Could you check a few things on this model? Use its own coordinates, in mm. Face numbers are marked on the shaded views. A direction names the side the tool comes from. Coordinates: 2 decimals unless noted, no trailing zeros. Loops run counter-clockwise (first coordinate to the right, second up) from the corner with the lowest first, then second, coordinate; pieces in that order, holes last. Notation, with made-up numbers: (9.25, 84) -> (33.25, 84) arc R11 ccw to (33.25, 98) -> close; hole circle Ø8 at (31.5, -23.5). An arc over 180 degrees is marked (long way). One line per question, with ' | ' between items.
from build123d import *

# Parameters (mm, degrees)
SKETCH1_W                       = 9.5
SKETCH1_H                       = 3.26
BOSS_EXTRUDE1_DEPTH             = 11.42
BOSS_EXTRUDE3_REACH             = 14.475
BOSS_EXTRUDE3_DIRECTION_2_REACH = 14.475
FILLET1_R                       = 0.3
SKETCH4_R                       = 1.5
CUT_EXTRUDE1_DEPTH              = 16.081341077
FILLET2_R                       = 10


with BuildPart() as part:
    # Sketch1 → Boss-Extrude1 (new body)
    with BuildSketch(Plane.XY):
        Rectangle(SKETCH1_W, SKETCH1_H)
    extrude(amount=BOSS_EXTRUDE1_DEPTH)

    # Boss-Extrude3: up to this face of the body (flat: up to its plane)
    boss_extrude3_end = Plane(part.part.faces().sort_by_distance((-4.75, 0, 5.71))[0])
    # Sketch3 → Boss-Extrude3 (add, up to the picked face)
    with BuildSketch(Plane(origin=(0, 0, 0), x_dir=(0, 0, -1), z_dir=(1, 0, 0)), mode=Mode.PRIVATE) as boss_extrude3_sk1:
        with BuildLine():
            Line((0, -1.63), (5.2, -2.629157971))
            add(Edge.make_bspline(
                [(5.2, -2.629157971), (5.283052086, -2.547091023), (5.363844635, -2.459497383), (5.60978901, -2.164369944), (5.763042084, -1.936211317), (6.019426683, -1.436050674), (6.122353138, -1.164082205), (6.261824898, -0.594664263), (6.298216306, -0.297392436), (6.298215992, 0.297396341), (6.26182427, 0.594668129), (6.122351908, 1.164085924), (6.019425166, 1.436054284), (5.763040038, 1.936214656), (5.609786724, 2.164373121), (5.363842902, 2.459499262), (5.283051196, 2.547091902), (5.2, 2.629157971)],
                knots=[0.163498388, 0.163498388, 0.163498388, 0.163498388, 0.204239042, 0.204239042, 0.29258857, 0.29258857, 0.380938098, 0.380938098, 0.469287626, 0.469287626, 0.557637154, 0.557637154, 0.645986682, 0.645986682, 0.73433621, 0.73433621, 0.77507641, 0.77507641, 0.77507641, 0.77507641], degree=3))
            Line((5.2, 2.629157971), (0, 1.63))
            Line((0, 1.63), (0, -1.63))
        make_face()
    boss_extrude3_tool1 = split(extrude(boss_extrude3_sk1.sketch, amount=-BOSS_EXTRUDE3_REACH, mode=Mode.PRIVATE), bisect_by=boss_extrude3_end, keep=Keep.BOTH, mode=Mode.PRIVATE)
    add(boss_extrude3_tool1.solids().sort_by(Axis((0, 0, -3.236322), (-1, 0, 0)))[0])

    # Boss-Extrude3 direction 2: up to this face of the body (flat: up to its plane)
    boss_extrude3_direction_2_end = Plane(part.part.faces().sort_by_distance((4.75, 0, 5.71))[0])
    # Sketch3 → Boss-Extrude3 direction 2 (add, up to the picked face)
    with BuildSketch(Plane(origin=(0, 0, 0), x_dir=(0, 0, -1), z_dir=(1, 0, 0)), mode=Mode.PRIVATE) as boss_extrude3_direction_2_sk1:
        with BuildLine():
            Line((0, -1.63), (5.2, -2.629157971))
            add(Edge.make_bspline(
                [(5.2, -2.629157971), (5.283052086, -2.547091023), (5.363844635, -2.459497383), (5.60978901, -2.164369944), (5.763042084, -1.936211317), (6.019426683, -1.436050674), (6.122353138, -1.164082205), (6.261824898, -0.594664263), (6.298216306, -0.297392436), (6.298215992, 0.297396341), (6.26182427, 0.594668129), (6.122351908, 1.164085924), (6.019425166, 1.436054284), (5.763040038, 1.936214656), (5.609786724, 2.164373121), (5.363842902, 2.459499262), (5.283051196, 2.547091902), (5.2, 2.629157971)],
                knots=[0.163498388, 0.163498388, 0.163498388, 0.163498388, 0.204239042, 0.204239042, 0.29258857, 0.29258857, 0.380938098, 0.380938098, 0.469287626, 0.469287626, 0.557637154, 0.557637154, 0.645986682, 0.645986682, 0.73433621, 0.73433621, 0.77507641, 0.77507641, 0.77507641, 0.77507641], degree=3))
            Line((5.2, 2.629157971), (0, 1.63))
            Line((0, 1.63), (0, -1.63))
        make_face()
    boss_extrude3_direction_2_tool1 = split(extrude(boss_extrude3_direction_2_sk1.sketch, amount=BOSS_EXTRUDE3_DIRECTION_2_REACH, mode=Mode.PRIVATE), bisect_by=boss_extrude3_direction_2_end, keep=Keep.BOTH, mode=Mode.PRIVATE)
    add(boss_extrude3_direction_2_tool1.solids().sort_by(Axis((0, 0, -3.236322), (1, 0, 0)))[0])

    # Fillet1
    fillet1_edges = [part.edges().sort_by_distance(p)[0] for p in [
        (2.375, 2.629157971, -5.2),
        (2.375, -2.629157971, -5.2),
    ]]
    fillet(fillet1_edges, radius=FILLET1_R)

    # Sketch4 → Cut-Extrude1 (cut, through all)
    with BuildSketch(Plane(origin=(4.75, 0, 0), x_dir=(0, 0, -1), z_dir=(1, 0, 0))):
        with Locations((3.698216149, 0)):
            Circle(SKETCH4_R)
    extrude(amount=-CUT_EXTRUDE1_DEPTH, mode=Mode.SUBTRACT)

    # Fillet2
    fillet2_edges = [part.edges().sort_by_distance(p)[0] for p in [
        (0, 1.63, 0),
        (0, -1.63, 0),
    ]]
    fillet(fillet2_edges, radius=FILLET2_R)


solid = part.part
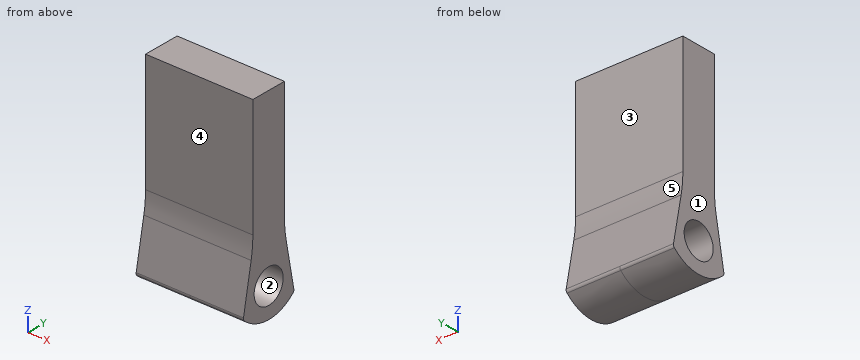
1) I'm going to push flat-ended pins straight in: pin 1 Ø1 at (x, z) = (1.5, 2) entering from -Y; pin 2 Ø1.8 at (y, z) = (0, -3.7) entering from -X (3 decimals). Where does each tip first touch, or does it pass through?
Data:
pin 1: y = -1.63 | pin 2: through
2) We'd pull the mould along Y, two halves only. Please class the marked faces 1, 2 and 3: pulls with the +Y half, pulls with the -Y half, needs draft (parallel to the pull), parting line crosses it, or undercut.
Data:
face 1: needs draft | face 2: undercut | face 3: pulls with the +Y half
3) On a 3-axis mill with a long thin cutter (end or side, diameter ignored), from which of +Z, -Z, +X, -X, +Y, -Y can I reach the whole of each face in a straight line? I mean the marked faces 4 and 5. Say none if no direction works.
Data:
face 4: +Z, +X, -X, -Y | face 5: +Z, +X, -X, +Y
4) If we section it at B-B on z = -0.75: Please give me the cut outline in (x, y), and give its area (3 significant figures).
Data:
outline: (-4.75, -1.78) -> (4.75, -1.78) -> (4.75, 1.78) -> (-4.75, 1.78) -> close | area: 33.7 mm²
5) If we section it at A-A on z = 9.5: Please give me the cut outline in (x, y).
Data:
outline: (-4.75, -1.63) -> (4.75, -1.63) -> (4.75, 1.63) -> (-4.75, 1.63) -> close
6) I need wall thicknesses on line 1 along Y through (x, z) = (-0.25, 4.25); line 2 along Y through (x, z) = (0, -3); line 3 along Z through (x, y) = (-2, -0.5). Which ranges of each line are inside material? Lowest first, please. Write a range as from..to.
Data:
line 1: -1.63..1.63 | line 2: -2.21..-1.33, 1.33..2.21 | line 3: -6.26..-5.11, -2.28..11.42
